Build history of the part. All positions in model axes, mm. Face numbers are marked on the shaded views. A direction names the side the tool comes from. Coordinates: 2 decimals unless noted, no trailing zeros. Write each loop counter-clockwise with the first axis right and the second up, starting at its lowest first coordinate (ties: lowest second). Pieces come first, ordered by that corner, then holes.
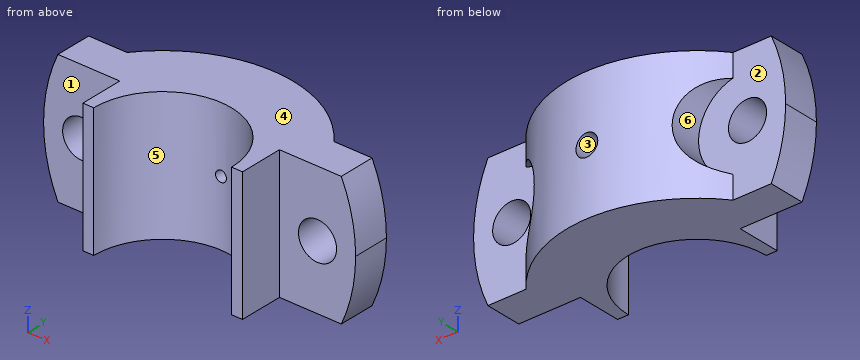
from build123d import *

# Parameters (mm, degrees)
BOSS_EXTRUDE1_DEPTH      = 36
CUT_EXTRUDE1_DEPTH       = 36
SKETCH3_R                = 12
CUT_EXTRUDE10_DEPTH      = 61.241181927
SKETCH10_R               = 3
CUT_EXTRUDE12_DEPTH      = 10
CUT_EXTRUDE13_DEPTH      = 61.241181987
CUT_EXTRUDE13_DEPTH_BACK = 61.241181987
SKETCH11_R               = 1.5
SKETCH9_R                = 5.25
CUT_EXTRUDE14_DEPTH      = 10


with BuildPart() as part:
    # Sketch1 → Boss-Extrude1 (new body)
    with BuildSketch(Plane.XY):
        with BuildLine():
            Line((-22, 0), (-19, 0))
            ThreePointArc((-19, 0), (0, 19), (19, 0))
            Line((19, 0), (22, 0))
            Line((22, 0), (22, 12))
            Line((22, 12), (43, 12))
            Line((43, 12), (43, 22))
            Line((43, 22), (28.495613698, 22))
            ThreePointArc((28.495613698, 22), (0, 36), (-28.495613698, 22))
            Line((-28.495613698, 22), (-43, 22))
            Line((-43, 22), (-43, 12))
            Line((-43, 12), (-22, 12))
            Line((-22, 12), (-22, 0))
        make_face()
    extrude(amount=-BOSS_EXTRUDE1_DEPTH)

    # Sketch2 → Cut-Extrude1 (cut)
    with BuildSketch(Plane(origin=(0, 22, 0), x_dir=(1, 0, 0), z_dir=(0, 1, 0))):
        with BuildLine():
            Line((-39.05124838, 36), (-43, 36))
            Line((-43, 36), (-43, 18))
            ThreePointArc((-43, 18), (-42.001212365, 27.214019744), (-39.05124838, 36))
        make_face()
        with BuildLine():
            ThreePointArc((-39.05124838, 0), (-42.001212365, 8.785980256), (-43, 18))
            Line((-43, 18), (-43, 0))
            Line((-43, 0), (-39.05124838, 0))
        make_face()
        with BuildLine():
            Line((43, 36), (39.05124838, 36))
            ThreePointArc((39.05124838, 36), (42.001212365, 27.214019744), (43, 18))
            Line((43, 18), (43, 36))
        make_face()
        with BuildLine():
            Line((43, 0), (43, 18))
            ThreePointArc((43, 18), (42.001212365, 8.785980256), (39.05124838, 0))
            Line((39.05124838, 0), (43, 0))
        make_face()
    extrude(amount=-CUT_EXTRUDE1_DEPTH, mode=Mode.SUBTRACT)

    # Sketch3 → Cut-Extrude10 (cut, through all)
    with BuildSketch(Plane(origin=(0, 22, 0), x_dir=(1, 0, 0), z_dir=(0, 1, 0))):
        with Locations((-31, 18)):
            Circle(SKETCH3_R)
        with Locations((31, 18)):
            Circle(SKETCH3_R)
    extrude(amount=CUT_EXTRUDE10_DEPTH, mode=Mode.SUBTRACT)

    # Sketch10 → Cut-Extrude12 (cut)
    with BuildSketch(Plane(origin=(0, 36, 0), x_dir=(1, 0, 0), z_dir=(0, 1, 0))):
        with Locations(Location((0, 18, 0), (0, 0, 180))):
            Circle(SKETCH10_R)
    extrude(amount=-CUT_EXTRUDE12_DEPTH, mode=Mode.SUBTRACT)

    # Sketch11 → Cut-Extrude13 (cut, two sides: drawn at the far end of the back side and taken through both)
    with BuildSketch(Plane(origin=(0, 22, 0), x_dir=(1, 0, 0), z_dir=(0, 1, 0)).offset(-CUT_EXTRUDE13_DEPTH_BACK)):
        with Locations(Location((0, 18, 0), (0, 0, 270))):
            Circle(SKETCH11_R)
    extrude(amount=CUT_EXTRUDE13_DEPTH + CUT_EXTRUDE13_DEPTH_BACK, mode=Mode.SUBTRACT)

    # Sketch9 → Cut-Extrude14 (cut)
    with BuildSketch(Plane(origin=(0, 22, 0), x_dir=(1, 0, 0), z_dir=(0, 1, 0))):
        with Locations(Location((-32.500715047, 18.084858078, 0), (0, 0, 270))):
            Circle(SKETCH9_R)
        with Locations(Location((32.499093077, 18.242794562, 0), (0, 0, 270))):
            Circle(SKETCH9_R)
    extrude(amount=-CUT_EXTRUDE14_DEPTH, mode=Mode.SUBTRACT)


solid = part.part
(1) Slice it at D-D, the plane y = 23.5. List the corners of the cut face in (x, z), and give its area (3 significant figures).
(2) Probe L1, parallel to X at y = 21.5, z = -18; L2, parallel to X at y = 24, z = -18; L3, parallel to X at y = 19.5, z = -14. List the from-to ranges inside material, lowest first.
(3) Slice it at C-C, the plane z = -32. List the corners of the cut face in (x, y).
(4) Two-plate mould, pull along X, no slides. Class the marked faces 4, 5 and 6: pulls with the +X half, pulls with the -X half, needs draft (parallel to the pull), parting line crosses it, or undercut.
(5) Flat gauge pins, fed straight in: P1, Ø5, axis at y = 22, z = -7.5, coming from the +X side; P2, Ø8, axis at y = 27.5, z = -4, coming from the -X side; P3, Ø10, axis at y = 17, z = -14.5, coming from the +X side; P4, Ø8, axis at y = 17, z = -8.5, coming from the -X side. Where does each tip first touch, or does it go through?
(6) 3-axis set-ups, long thin cutter, end or side, ignore diameter. For the marked faces 1, 2 and 3: which of +Z, -Z, +X, -X, +Y, -Y reach the whole face in a straight line?
(7) Slice it at A-A, the plane x = 0. List the corners of the cut face in (y, z).
(8) Slice it at B-B, the plane y = 17. List the corners of the cut face in (x, z).
Results:
1. outline: (-27.27, -36) - (27.27, -36) - (27.27, -29.41) arc R12 cw to (27.27, -6.59) - (27.27, 0) - (-27.27, 0) - (-27.27, -6.59) arc R12 cw to (-27.27, -29.41) - close; hole circle Ø3 at (0, -18)
1. area: 1,680 mm2
2. L1: x = -43 to -37.75, -27.25 to -1.5, 1.5 to 27.25, 37.74 to 43
2. L2: x = -19 to -1.5, 1.5 to 19
2. L3: x = -42.81 to -35.8, -29.2 to 29.41, 35.59 to 42.81
3. outline: (-40.66, 12) - (-22, 12) - (-22, 0) - (-19, 0) arc R19 cw to (19, 0) - (22, 0) - (22, 12) - (40.66, 12) - (40.66, 22) - (28.5, 22) arc R36 ccw to (-28.5, 22) - (-40.66, 22) - close
4. face 4: needs draft
4. face 5: undercut
4. face 6: pulls with the -X half
5. P1: stops at x = 42.25
5. P2: stops at x = -27.27
5. P3: stops at x = 43
5. P4: stops at x = -42.65
6. face 1: +Z, -Z, -X, -Y
6. face 2: -X, +Y
6. face 3: +Y
7. outline: (19, -36) - (36, -36) - (36, -21) - (26, -21) - (26, -19.5) - (19, -19.5) - close; (19, -16.5) - (26, -16.5) - (26, -15) - (36, -15) - (36, 0) - (19, 0) - close
8. outline: (-39.05, -36) - (-8.49, -36) - (-8.49, 0) - (-39.05, 0) arc R43 ccw to start; (8.49, -36) - (39.05, -36) arc R43 ccw to (39.05, 0) - (8.49, 0) - close; hole circle Ø10.5 at (-32.5, -18.08); hole circle Ø10.5 at (32.5, -18.24)
